```python
from build123d import *

# Parameters (mm, degrees)
SKETCH003_W                   = 254
SKETCH003_H                   = 152.4
PAD001_DEPTH                  = 25.4
POCKET002_DEPTH               = 619.999755
POCKET003_DEPTH               = 4.318
POCKET002_MIRRORED002_2_DEPTH = 619.999755


with BuildPart() as part:
    # Sketch003 (on Face1 of ShapeBinder) → Pad001 (new body)
    with BuildSketch(Plane.XY.offset(25.4)):
        Rectangle(SKETCH003_W, SKETCH003_H)
    extrude(amount=PAD001_DEPTH)

    # Sketch004 (on Face1 of ShapeBinder) → Pocket002 (cut, through all)
    with BuildSketch(Plane.XY.offset(25.4)):
        with BuildLine():
            ThreePointArc((-95.6, 46.3), (-91.1, 50.8), (-95.6, 55.3))
            Line((-95.6, 55.3), (-127, 55.3))
            Line((-127, 55.3), (-127, 46.3))
            Line((-127, 46.3), (-95.6, 46.3))
        make_face()
    pocket002 = extrude(amount=POCKET002_DEPTH, mode=Mode.SUBTRACT)

    # Sketch005 (on Face1 of ShapeBinder) → Pocket003 (cut)
    with BuildSketch(Plane.XY.offset(25.4)):
        with BuildLine():
            Line((127, -12.7), (74.586888, -12.7))
            ThreePointArc((74.586888, 12.7), (-25.4, 0), (74.586888, -12.7))
            Line((74.586888, 12.7), (127, 12.7))
            Line((127, 12.7), (127, -12.7))
        make_face()
    extrude(amount=POCKET003_DEPTH, mode=Mode.SUBTRACT)

    # Sketch004 Mirrored002 2 → Pocket002 Mirrored002 2 (cut, through all)
    with BuildSketch(Plane(origin=(0, 0, 25.4), x_dir=(-1, 0, 0), z_dir=(0, 0, -1))):
        with BuildLine():
            ThreePointArc((-95.6, 46.3), (-91.1, 50.8), (-95.6, 55.3))
            Line((-95.6, 55.3), (-127, 55.3))
            Line((-127, 55.3), (-127, 46.3))
            Line((-127, 46.3), (-95.6, 46.3))
        make_face()
    pocket002_mirrored002_2 = extrude(amount=-POCKET002_MIRRORED002_2_DEPTH, mode=Mode.SUBTRACT)

    # Mirrored003: Pocket002, Pocket002 Mirrored002 2 across XZ
    add(pocket002.mirror(Plane.XZ), mode=Mode.SUBTRACT)
    add(pocket002_mirrored002_2.mirror(Plane.XZ), mode=Mode.SUBTRACT)


solid = part.part
```
Check sheet for the modelled part. Datum: model origin and axes. Units: mm. A direction names the side the tool comes from. Give positions to 0.01 mm unless a question says otherwise; leave off trailing zeros. Order: outer loops, then holes, each group sorted by start corner. A loop starts at its lowest first (then second) coordinate and runs counter-clockwise, first axis right, second up. Notation, with made-up numbers: (-40, 27) -> (17, 27) arc R21 cw to (17, 64) -> close; hole circle Ø3 at (24.25, 6.25). An arc over 180 degrees is marked (long way). Return JSON: item names as keys, results as strings.
1. Go/stop test with a flat-tipped pin: P1, Ø3, axis at x = 40.5, y = -28, coming from the -Z side. Record where the tip stops, or that it passes through.
From the geometry:
{"P1": "z = 29.72"}
2. Mould release check, pull along Y, two halves, no side actions. Record for faces 6 (the flat face through (-127, 66, 38)), 7 (the cylindrical face through (91.1, -50.7, 37.9)), 8 (the flat face through (111, 55.3, 38)): +Y half, -Y half, draft (parallel to the pull), parting line (faces both ways), or undercut.
From the geometry:
{"face 6": "draft", "face 7": "undercut", "face 8": "undercut"}
3. Cross-section at A-A, the plane x = 104.5. Record the cut outline in (y, z).
From the geometry:
{"outline": "(-76.2, 25.4) -> (-55.3, 25.4) -> (-55.3, 50.8) -> (-76.2, 50.8) -> close; (-46.3, 25.4) -> (-12.7, 25.4) -> (-12.7, 29.72) -> (12.7, 29.72) -> (12.7, 25.4) -> (46.3, 25.4) -> (46.3, 50.8) -> (-46.3, 50.8) -> close; (55.3, 25.4) -> (76.2, 25.4) -> (76.2, 50.8) -> (55.3, 50.8) -> close"}
4. Material ranges on probe 1 along Y at (x, z) = (102, 38.25); probe 2 along Y at (x, z) = (25.4, 28.8); probe 3 along X at (y, z) = (0, 27.9), recorded low to high. Write a range as [from, to].
From the geometry:
{"probe 1": "[-76.2, -55.3], [-46.3, 46.3], [55.3, 76.2]", "probe 2": "[-76.2, -50.8], [50.8, 76.2]", "probe 3": "[-127, -25.4]"}
5. Cross-section at B-B, the plane z = 44.75. Record the cut outline in (x, y), plus the area to 3 significant figures.
From the geometry:
{"outline": "(-127, -76.2) -> (127, -76.2) -> (127, -55.3) -> (95.6, -55.3) arc R4.5 cw to (95.6, -46.3) -> (127, -46.3) -> (127, 46.3) -> (95.6, 46.3) arc R4.5 cw to (95.6, 55.3) -> (127, 55.3) -> (127, 76.2) -> (-127, 76.2) -> (-127, 55.3) -> (-95.6, 55.3) arc R4.5 cw to (-95.6, 46.3) -> (-127, 46.3) -> (-127, -46.3) -> (-95.6, -46.3) arc R4.5 cw to (-95.6, -55.3) -> (-127, -55.3) -> close", "area": "37,500 mm^2"}
6. Cross-section at C-C, the plane y = 19.5. Record the cut outline in (x, z).
From the geometry:
{"outline": "(-127, 25.4) -> (-21.51, 25.4) -> (-21.51, 29.72) -> (72.31, 29.72) -> (72.31, 25.4) -> (127, 25.4) -> (127, 50.8) -> (-127, 50.8) -> close"}
7. Set-up check for faces 1 (the flat face through (112, 46.3, 38)), 2 (the flat face through (35, 1, 29.718)), 3 (the flat face through (-112, -46.3, 38)), 4 (the flat face through (127, 66, 38)), 5 (the flat face through (-127, -66, 38)): record each of +Z, -Z, +X, -X, +Y, -Y from which the full face is reachable in a straight line by a thin tool's end or side.
From the geometry:
{"face 1": "+Z, -Z, +X", "face 2": "-Z", "face 3": "+Z, -Z, -X", "face 4": "+Z, -Z, +X, +Y, -Y", "face 5": "+Z, -Z, -X, +Y, -Y"}
8. Cross-section at D-D, the plane x = -100.5. Record the cut outline in (y, z), plus the area to 3 significant figures.
From the geometry:
{"outline": "(-76.2, 25.4) -> (-55.3, 25.4) -> (-55.3, 50.8) -> (-76.2, 50.8) -> close; (-46.3, 25.4) -> (46.3, 25.4) -> (46.3, 50.8) -> (-46.3, 50.8) -> close; (55.3, 25.4) -> (76.2, 25.4) -> (76.2, 50.8) -> (55.3, 50.8) -> close", "area": "3,410 mm^2"}
